Source: three-view drawing plus pictorial views. Frame: mm from the lowest corner of the part. A direction names the side the tool comes from. Round coordinates to 2 decimals unless told otherwise and drop trailing zeros. Loops run counter-clockwise (first coordinate to the right, second up) from the corner with the lowest first, then second, coordinate; pieces in that order, holes last. Notation, with made-up numbers: (-28, -24.5) -> (4, -24.5) arc R21 cw to (4, 12.5) -> close; hole circle Ø6 at (-3, 64.5). An arc over 180 degrees is marked (long way). One line per question, with ' | ' between items. Start each with the question number.
Q1. Access query for the marked faces 1, 2 and 3. Directions: +Z, -Z, +X, -X, +Y, -Y. A direction counts if a zero-diameter tool reaches every point of the face in a straight line with its end or side. Return the directions, or none.
Q2. Cut plane C-C on y = 10. Return loops of the section in (x, z), and give its area (3 significant figures).
Q3. Mould query, pull axis Y, two halves, no side actions, for the marked faces 4, 5, 6 and 7. Classes: pulls with the +Y half, pulls with the -Y half, needs draft (parallel to the pull), parting line crosses it, or undercut.
Q4. Cut plane D-D on x = 65.5. Return loops of the section in (y, z).
Q5. Cut plane B-B on z = 5.5. Return loops of the section in (x, y), and give its area (3 significant figures).
Q6. Cut plane A-A on x = 89. Return loops of the section in (y, z), and give its area (3 significant figures).
Q7. Contact query for flat-ended pins moving along their axis: P1, Ø9.5, axis at y = 21.5, z = 5.5, coming from the -X side; P2, Ø8, axis at y = 10.5, z = 18.5, coming from the -X side; P3, Ø15, axis at x = 40, y = 18.5, coming from the +Z side. Output: stop coordinate, or through.
Q8. Material intervals for L1, parallel to Y at x = 13, z = 5; L2, parallel to Z at x = 45, y = 20; L3, parallel to X at y = 25.5, z = 22, sorted ascending.
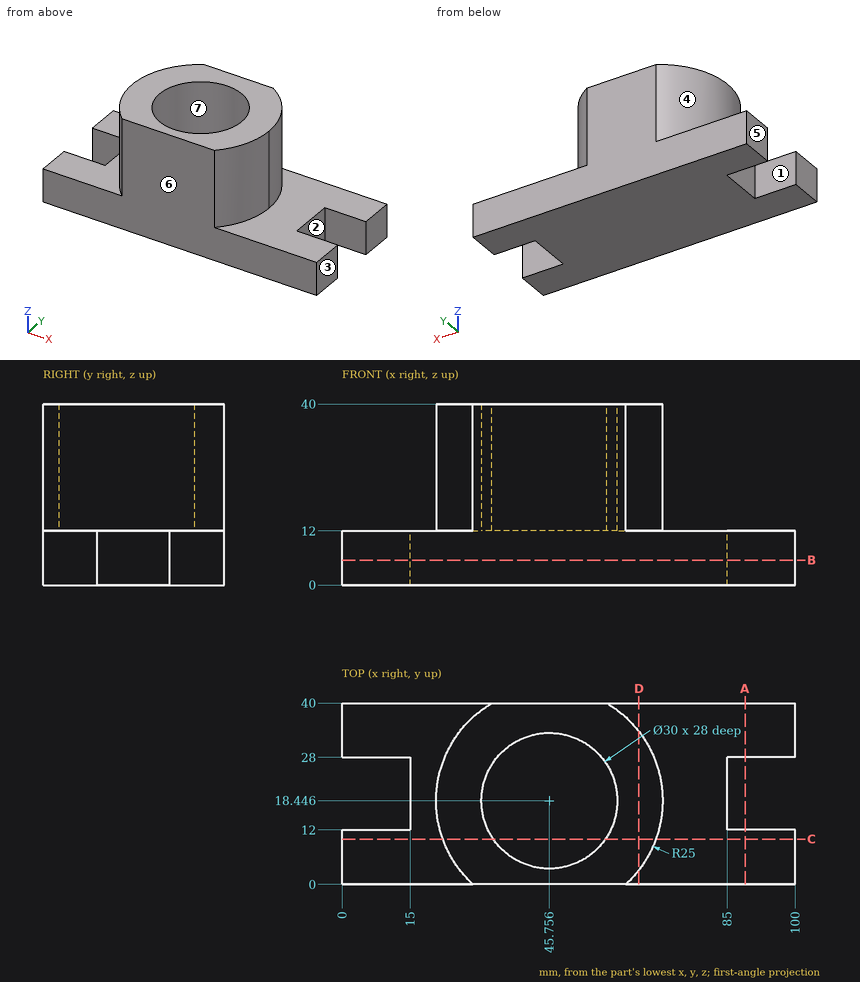
Results:
1) face 1: +Z, -Z, -X | face 2: +Z, -Z, +X | face 3: +Z, -Z, +X, +Y, -Y
2) outline: (0, 0) -> (100, 0) -> (100, 12) -> (69.29, 12) -> (69.29, 40) -> (58.15, 40) -> (58.15, 12) -> (33.36, 12) -> (33.36, 40) -> (22.23, 40) -> (22.23, 12) -> (0, 12) -> close | area: 1,820 mm^2
3) face 4: parting line crosses it | face 5: needs draft | face 6: pulls with the -Y half | face 7: undercut
4) outline: (0, 0) -> (40, 0) -> (40, 12) -> (33.78, 12) -> (33.78, 40) -> (3.11, 40) -> (3.11, 12) -> (0, 12) -> close
5) outline: (0, 0) -> (100, 0) -> (100, 12) -> (85, 12) -> (85, 28) -> (100, 28) -> (100, 40) -> (0, 40) -> (0, 28) -> (15, 28) -> (15, 12) -> (0, 12) -> close | area: 3,520 mm^2
6) outline: (0, 0) -> (12, 0) -> (12, 12) -> (0, 12) -> close; (28, 0) -> (40, 0) -> (40, 12) -> (28, 12) -> close | area: 288 mm^2
7) P1: x = 15 | P2: x = 21.07 | P3: z = 12
8) L1: 0 to 12, 28 to 40 | L2: 0 to 12 | L3: 21.77 to 32.52, 58.99 to 69.74
